Autodesk Inventor part; units mm, degrees
ref_plane "YZ Plane" through (0, 0, 0) normal (1, 0, 0) x (0, 1, 0)
ref_plane "XZ Plane" through (0, 0, 0) normal (0, 1, 0) x (-1, 0, 0)
ref_plane "XY Plane" through (0, 0, 0) normal (0, 0, 1) x (1, 0, 0)
sketch "Baza" plane through (0, 0, 0) normal (0, 1, 0) x (-1, 0, 0)
  line L0 (30, 30) -> (-30, 30) construction
  line L1 (-30, 30) -> (-30, -30) construction
  line L2 (-30, -30) -> (30, -30) construction
  line L3 (30, -30) -> (30, 30) construction
  line L4 (30, 30) -> (-30, -30) construction
  line L5 (-30, 30) -> (30, -30) construction
  circle A0 centre (30, -30) radius 3
  circle A1 centre (30, 30) radius 3
  circle A2 centre (-30, 30) radius 3
  circle A3 centre (-30, -30) radius 3
  line L6 (37.5, 37.5) -> (-37.5, 37.5)
  line L7 (-37.5, 37.5) -> (-37.5, -37.5)
  line L8 (-37.5, -37.5) -> (37.5, -37.5)
  line L9 (37.5, -37.5) -> (37.5, 37.5)
  line L10 (37.5, 37.5) -> (-37.5, -37.5) construction
  line L11 (-37.5, 37.5) -> (37.5, -37.5) construction
  line L12 (10.475, 26.2) -> (-10.475, 26.2) construction
  line L13 (-10.475, 26.2) -> (-10.475, -26.2) construction
  line L14 (-10.475, -26.2) -> (10.475, -26.2) construction
  line L15 (10.475, -26.2) -> (10.475, 26.2) construction
  line L16 (10.475, 26.2) -> (-10.475, -26.2) construction
  line L17 (-10.475, 26.2) -> (10.475, -26.2) construction
  circle A4 centre (10.475, 26.2) radius 1.25
  circle A5 centre (-10.475, 26.2) radius 1.25
  circle A6 centre (-10.475, -26.2) radius 1.25
  circle A7 centre (10.475, -26.2) radius 1.25
  line L18 (12, 16) -> (-12, 16)
  line L19 (-12, 16) -> (-12, -16)
  line L20 (-12, -16) -> (12, -16)
  line L21 (12, -16) -> (12, 16)
  line L22 (12, 16) -> (-12, -16) construction
  line L23 (-12, 16) -> (12, -16) construction
  circle A8 centre (16.413, 21.1229) radius 1.6
  circle A9 centre (-16.413, -21.1229) radius 1.6
  point P0 (0, 0)
  dimension "d0" = 60
  dimension "d1" = 6
  dimension "d2" = 75
  dimension "d3" = 20.95
  dimension "d4" = 52.4
  dimension "d5" = 2.5
  dimension "d6" = 24
  dimension "d7" = 32
  dimension "d12" = 3.2
  dimension "d20" = 5.938
  dimension "d21" = 5.0771
  dimension "d22" = 5.938
  dimension "d23" = 5.0771
extrude "Wyciągnięcie proste1" add sketch "Baza" along normal blind 15
sketch "Szkic2" plane through (0, 15, 0) normal (0, 1, 0) x (1, 0, 0)
  line L0 (37.5, -37.5) -> (37.5, 37.5)
  line L1 (37.5, 37.5) -> (-37.5, 37.5)
  line L2 (-37.5, 37.5) -> (-37.5, -37.5)
  line L3 (-37.5, -37.5) -> (37.5, -37.5)
  circle A0 centre (16.413, 21.1229) radius 1.6
  circle A1 centre (-10.475, 26.2) radius 1.25
  circle A2 centre (10.475, 26.2) radius 1.25
  circle A3 centre (10.475, -26.2) radius 1.25
  circle A4 centre (-10.475, -26.2) radius 1.25
  circle A5 centre (30, 30) radius 3
  circle A6 centre (30, -30) radius 3
  circle A7 centre (-30, -30) radius 3
  circle A8 centre (-30, 30) radius 3
  circle A9 centre (-16.413, -21.1229) radius 1.6
  line L4 (-12, -16) -> (-12, 16)
  line L5 (-12, 16) -> (12, 16)
  line L6 (12, 16) -> (12, -16)
  line L7 (12, -16) -> (-12, -16)
  line L8 (-12, -16) -> (-12, 16)
  point P0 (0, 0)
sketch "Szkic3" plane through (0, 15, 0) normal (0, 1, 0) x (1, 0, 0)
  line L0 (25, -24.5) -> (-25, -24.5)
  line L1 (-25, -24.5) -> (-25, 24.5)
  line L2 (-25, 24.5) -> (25, 24.5)
  line L3 (25, 24.5) -> (25, -24.5)
  line L4 (25, -24.5) -> (-25, 24.5) construction
  line L5 (-25, -24.5) -> (25, 24.5) construction
  point P0 (0, 0)
  dimension "d16" = 49
  dimension "d17" = 50
extrude "Wyciągnięcie proste2" cut sketch "Szkic3" against normal blind 9.7
sketch "Szkic4" plane through (0, 15, 0) normal (0, 1, 0) x (1, 0, 0)
  line L0 (37.5, 37.5) -> (-37.5, 37.5)
  line L1 (-37.5, -37.5) -> (37.5, -37.5)
  line L2 (-25, 37.5) -> (-18.475, 37.5)
  line L3 (-18.475, 37.5) -> (-18.475, -37.5)
  line L4 (-18.475, -37.5) -> (-25, -37.5)
  line L5 (-25, -37.5) -> (-25, 37.5)
  circle A0 centre (-10.475, 26.2) radius 1.25
  line L6 (-25, -24.5) -> (-25, 24.5)
  point P0 (0, 0)
  dimension "d24" = 8
extrude "Wyciągnięcie proste3" cut sketch "Szkic4" against normal blind 8 contours L3 L1 L5 L0
properties part number "dmd_cnc"
Read the model definition and answer for the solid it produces. Units are mm, in the model's axes. A direction names the side the tool comes from. Coordinates: 2 decimals unless noted, no trailing zeros. Loops run counter-clockwise (first coordinate to the right, second up) from the corner with the lowest first, then second, coordinate; pieces in that order, holes last. Notation, with made-up numbers: (13, 2) -> (20, 2) arc R16 ccw to (20, 18) -> close; hole circle Ø8 at (49, 50.25). An arc over 180 degrees is marked (long way). Return JSON: item names as keys, results as strings.
Item 1: For a pull along Z with two mould halves and no side action, classify faces 6 (the flat face through (-18.475, 11, 31)), 7 (the flat face through (12, 3, 0)), 8 (the flat face through (-1, 7, 37.5)) as +Z half, -Z half, draft (parallel to the pull), parting line (faces both ways), or undercut.
Answers:
{"face 6": "draft", "face 7": "undercut", "face 8": "+Z half"}
Item 2: Find section C-C (x = 30). Determine the outline of the cut face in (y, z), plus the area to 3 significant figures.
Answers:
{"outline": "(0, -37.5) -> (15, -37.5) -> (15, -33) -> (0, -33) -> close; (0, -27) -> (15, -27) -> (15, 27) -> (0, 27) -> close; (0, 33) -> (15, 33) -> (15, 37.5) -> (0, 37.5) -> close", "area": "945 mm2"}
Item 3: For faces 1 (the flat face through (-16, 0, 1)), 2 (the flat face through (0, 3, 16)), 3 (the flat face through (-25, 10, 1)), 4 (the flat face through (-22, 7, 31)), 5 (the flat face through (-31, 15, 1)), determine the directions among +Z, -Z, +X, -X, +Y, -Y from which every point of the face is accessible in a straight line to the end or side of a thin tool.
Answers:
{"face 1": "+Z, -Z, +X, -X, -Y", "face 2": "+Y, -Y", "face 3": "+Y", "face 4": "+Z, -Z, +Y", "face 5": "+Z, -Z, +X, -X, +Y"}
Item 4: Find section A-A (y = 13.75). Count the separate pieces of the cut face and the enclosed holes in it, plus the area to 3 significant figures.
Answers:
{"separate pieces": "2", "enclosed holes": "8", "area": "2,870 mm2"}
Item 5: Find the intervals of material crossed by probe 1 along Z at (x, y) = (30, 10.5); probe 2 along X at (y, z) = (6.25, -26); probe 3 along X at (y, z) = (11.5, -2), in increasing order.
Answers:
{"probe 1": "z = -37.5 to -33, -27 to 27, 33 to 37.5", "probe 2": "x = -37.5 to -11.71, -9.24 to 9.24, 11.71 to 37.5", "probe 3": "x = -37.5 to -25, 25 to 37.5"}
Item 6: Find section B-B (z = -30). Determine the outline of the cut face in (x, y) (3 decimals).
Answers:
{"outline": "(-37.5, 0) -> (-33, 0) -> (-33, 15) -> (-37.5, 15) -> close; (-27, 0) -> (27, 0) -> (27, 15) -> (-18.475, 15) -> (-18.475, 7) -> (-25, 7) -> (-25, 15) -> (-27, 15) -> close; (33, 0) -> (37.5, 0) -> (37.5, 15) -> (33, 15) -> close"}
Item 7: Flat-ended cylindrical pins translate along their axes: P1, Ø2, axis at x = 19, z = -15, coming from the -Y side; P2, Ø14.5, axis at x = 9, z = 8, coming from the +Y side; P3, Ø2, axis at x = -22, z = 31.5, coming from the +Y side. Find the tip coordinate at first contact, or state that the pin passes through.
Answers:
{"P1": "stops at y = 0", "P2": "stops at y = 5.3", "P3": "stops at y = 7"}
